from build123d import *

# Parameters (mm, degrees)
SKETCH1_W          = 203.2
SKETCH1_H          = 203.2
BASE_FLANGE1_DEPTH = 3.175
SKETCH6_R          = 9.5631
SKETCH6_R_2        = 14.2621
SKETCH6_R_3        = 2.032
CUT_EXTRUDE1_DEPTH = 3.175


# Sheet-metal steps are written as plain solids
with BuildPart() as part:
    # Sketch1 → Base-Flange1 (new body)
    with BuildSketch(Plane(origin=(0, 0, 0), x_dir=(0, 0, -1), z_dir=(1, 0, 0))):
        Rectangle(SKETCH1_W, SKETCH1_H)
    extrude(amount=-BASE_FLANGE1_DEPTH)

    # Sketch6 → Cut-Extrude1 (cut)
    with BuildSketch(Plane(origin=(0, 0, 0), x_dir=(0, 0, -1), z_dir=(1, 0, 0))):
        with Locations((-34.6218707, 40.676977416)):
            Circle(SKETCH6_R)
        with Locations((34.6218707, 40.676977416)):
            Circle(SKETCH6_R)
        with Locations((-34.6218707, -40.676977416)):
            Circle(SKETCH6_R)
        with Locations((34.6218707, -40.676977416)):
            Circle(SKETCH6_R)
        Circle(SKETCH6_R_2)
        with Locations((-34.6218707, 66.076977416)):
            Circle(SKETCH6_R_3)
        with Locations((-34.6218707, 15.276977416)):
            Circle(SKETCH6_R_3)
        with Locations((-60.0218707, 40.676977416)):
            Circle(SKETCH6_R_3)
        with Locations((-9.2218707, 40.676977416)):
            Circle(SKETCH6_R_3)
        with Locations(Location((34.6218707, 15.276977416, 0), (0, 0, 180))):
            Circle(SKETCH6_R_3)
        with Locations(Location((60.0218707, 40.676977416, 0), (0, 0, 180))):
            Circle(SKETCH6_R_3)
        with Locations(Location((9.2218707, 40.676977416, 0), (0, 0, 180))):
            Circle(SKETCH6_R_3)
        with Locations(Location((34.6218707, 66.076977416, 0), (0, 0, 180))):
            Circle(SKETCH6_R_3)
        with Locations((34.6218707, -15.276977416)):
            Circle(SKETCH6_R_3)
        with Locations((60.0218707, -40.676977416)):
            Circle(SKETCH6_R_3)
        with Locations((34.6218707, -66.076977416)):
            Circle(SKETCH6_R_3)
        with Locations((9.2218707, -40.676977416)):
            Circle(SKETCH6_R_3)
        with Locations(Location((-9.2218707, -40.676977416, 0), (0, 0, 180))):
            Circle(SKETCH6_R_3)
        with Locations(Location((-34.6218707, -15.276977416, 0), (0, 0, 180))):
            Circle(SKETCH6_R_3)
        with Locations(Location((-60.0218707, -40.676977416, 0), (0, 0, 180))):
            Circle(SKETCH6_R_3)
        with Locations(Location((-34.6218707, -66.076977416, 0), (0, 0, 180))):
            Circle(SKETCH6_R_3)
    extrude(amount=-CUT_EXTRUDE1_DEPTH, mode=Mode.SUBTRACT)


solid = part.part
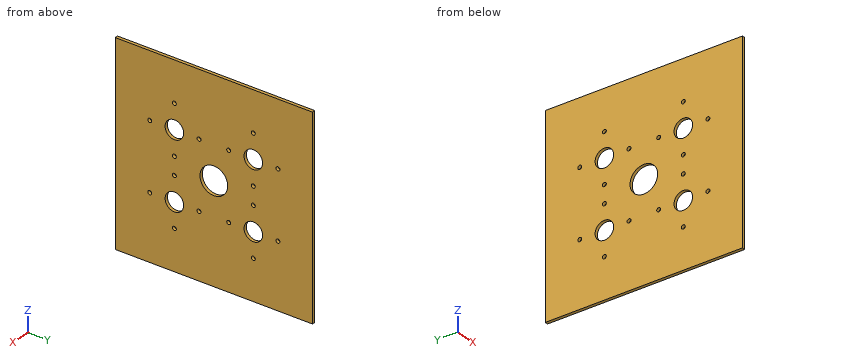
The model under review builds one solid part; all positions refer to its coordinate system, in mm. Round coordinates to 2 decimals unless told otherwise and drop trailing zeros. Loops run counter-clockwise (first coordinate to the right, second up) from the corner with the lowest first, then second, coordinate; pieces in that order, holes last. Notation, with made-up numbers: (-19, 76) -> (35, 76) arc R30 ccw to (35, 108) -> close; hole circle Ø4 at (-2, -6). An arc over 180 degrees is marked (long way). Answer as CSV lines item,"result".
1) Add section A-A on y = 0. Write out the cut boundary in (x, z) (3 decimals), plus the area to 3 significant figures.
Geometry results:
outline,"(-3.175, -101.6) -> (0, -101.6) -> (0, -14.262) -> (-3.175, -14.262) -> close; (-3.175, 14.262) -> (0, 14.262) -> (0, 101.6) -> (-3.175, 101.6) -> close"
area,"555 mm²"
2) Add section C-C on x = -0.9. State how many separate pieces and enclosed holes the cut face has, plus the area to 3 significant figures.
Geometry results:
separate pieces,"1"
enclosed holes,"21"
area,"39,300 mm²"
3) To check wall thickness, follow line 1 along Z through (x, y) = (-0.55, -1); line 2 along Y through (x, z) = (-2.5, -30.5); line 3 along Y through (x, z) = (-2.9, 28). State the ranges of each line that lie inside material, in increasing order. Write a range as from..to.
Geometry results:
line 1,"z = -101.6..-14.23, 14.23..101.6"
line 2,"y = -101.6..-49.31, -32.05..32.05, 49.31..101.6"
line 3,"y = -101.6..-47.58, -33.78..33.78, 47.58..101.6"
4) For P1, Ø17, axis at y = 40.68, z = -34.62, coming from the -X side; P2, Ø6.5, axis at y = -40.68, z = -60.02, coming from the +X side, all flat-tipped, find the tip position at first contact; note any pin that passes through.
Geometry results:
P1,"passes through"
P2,"stops at x = 0"
